from build123d import *

# Parameters (mm, degrees)
CROQUIS1_W                         = 32
CROQUIS1_H                         = 46
SALIENTE_EXTRUIR1_DEPTH            = 15
CROQUIS2_R                         = 7.5
SALIENTE_EXTRUIR2_DEPTH            = 30.8
CROQUIS3_R                         = 2.5
CROQUIS3_R_2                       = 1
CROQUIS3_R_3                       = 2.25
CROQUIS3_R_4                       = 6.25
CROQUIS3_R_5                       = 4
CROQUIS3_R_6                       = 3.958709401
CROQUIS3_R_7                       = 3.163808824
SALIENTE_EXTRUIR3_DEPTH            = 1
CORTAR_EXTRUIR1_START              = -10
CROQUIS3_3_R                       = 3.163808824
CORTAR_EXTRUIR1_DEPTH              = 10
TALADRO_DE_MARGEN_PARA_M1_41_D     = 1.8
TALADRO_DE_MARGEN_PARA_M1_41_DEPTH = 3
TALADRO_DE_MARGEN_PARA_M1_41_TIP   = 0.540774557


with BuildPart() as part:
    # Croquis1 → Saliente-Extruir1 (new body)
    with BuildSketch(Plane(origin=(0, 0, 0), x_dir=(1, 0, 0), z_dir=(0, 1, 0))):
        Rectangle(CROQUIS1_W, CROQUIS1_H)
    extrude(amount=SALIENTE_EXTRUIR1_DEPTH)

    # Croquis2 → Saliente-Extruir2 (add)
    with BuildSketch(Plane.XY.offset(23)):
        with Locations((8.5, 7.5)):
            Circle(CROQUIS2_R)
    extrude(amount=SALIENTE_EXTRUIR2_DEPTH)

    # Croquis3 → Saliente-Extruir3 (add)
    # profile 1 of 8: a face of its own
    with BuildSketch(Plane(origin=(0, 15, 0), x_dir=(1, 0, 0), z_dir=(0, 1, 0))):
        with Locations(Location((-11, 18, 0), (0, 0, 90))):
            Circle(CROQUIS3_R)
        with Locations(Location((-11, 18, 0), (0, 0, 270))):
            Circle(CROQUIS3_R_2, mode=Mode.SUBTRACT)
    # profile 2 of 8: a face of its own
    with BuildSketch(Plane(origin=(0, 15, 0), x_dir=(1, 0, 0), z_dir=(0, 1, 0))):
        with Locations(Location((11, 18, 0), (0, 0, 270))):
            Circle(CROQUIS3_R)
        with Locations(Location((11, 18, 0), (0, 0, 90))):
            Circle(CROQUIS3_R_2, mode=Mode.SUBTRACT)
    # profile 3 of 8: a face of its own
    with BuildSketch(Plane(origin=(0, 15, 0), x_dir=(1, 0, 0), z_dir=(0, 1, 0))):
        with Locations(Location((-5, -1, 0), (0, 0, 90))):
            Circle(CROQUIS3_R_3)
    # profile 4 of 8: a face of its own
    with BuildSketch(Plane(origin=(0, 15, 0), x_dir=(1, 0, 0), z_dir=(0, 1, 0))):
        with Locations(Location((5, -1, 0), (0, 0, 270))):
            Circle(CROQUIS3_R_3)
    # profile 5 of 8: a face of its own
    with BuildSketch(Plane(origin=(0, 15, 0), x_dir=(1, 0, 0), z_dir=(0, 1, 0))):
        with Locations(Location((-11, -18, 0), (0, 0, 270))):
            Circle(CROQUIS3_R)
        with Locations(Location((-11, -18, 0), (0, 0, 90))):
            Circle(CROQUIS3_R_2, mode=Mode.SUBTRACT)
    # profile 6 of 8: a face of its own
    with BuildSketch(Plane(origin=(0, 15, 0), x_dir=(1, 0, 0), z_dir=(0, 1, 0))):
        with Locations(Location((11, -18, 0), (0, 0, 90))):
            Circle(CROQUIS3_R)
        with Locations(Location((11, -18, 0), (0, 0, 270))):
            Circle(CROQUIS3_R_2, mode=Mode.SUBTRACT)
    # profile 7 of 8: a face of its own
    with BuildSketch(Plane(origin=(0, 15, 0), x_dir=(1, 0, 0), z_dir=(0, 1, 0))):
        with Locations(Location((0, 10.5, 0), (0, 0, 90))):
            Circle(CROQUIS3_R_4)
        with Locations(Location((0, 10.5, 0), (0, 0, 270))):
            Circle(CROQUIS3_R_5, mode=Mode.SUBTRACT)
    # profile 8 of 8: a face of its own
    with BuildSketch(Plane(origin=(0, 15, 0), x_dir=(1, 0, 0), z_dir=(0, 1, 0))):
        with Locations(Location((0, 10.5, 0), (0, 0, 90))):
            Circle(CROQUIS3_R_6)
        with Locations(Location((0, 10.5, 0), (0, 0, 270))):
            Circle(CROQUIS3_R_7, mode=Mode.SUBTRACT)
    extrude(amount=SALIENTE_EXTRUIR3_DEPTH)

    # Croquis3_3 → Cortar-Extruir1 (cut)
    with BuildSketch(Plane(origin=(0, 15, 0), x_dir=(1, 0, 0), z_dir=(0, 1, 0)).offset(CORTAR_EXTRUIR1_START)):
        with Locations(Location((0, 10.5, 0), (0, 0, 270))):
            Circle(CROQUIS3_3_R)
    extrude(amount=CORTAR_EXTRUIR1_DEPTH, mode=Mode.SUBTRACT)

    # Taladro de margen para M1.41
    with Locations(Plane(origin=(0, 15, 0), x_dir=(1, 0, 0), z_dir=(0, 1, 0))):
        with Locations((-14.5, 21.5), (14.5, 21.5), (-14.5, -21.5), (14.5, -21.5)):
            Hole(TALADRO_DE_MARGEN_PARA_M1_41_D / 2, depth=TALADRO_DE_MARGEN_PARA_M1_41_DEPTH)
            with Locations((0, 0, -(TALADRO_DE_MARGEN_PARA_M1_41_DEPTH + TALADRO_DE_MARGEN_PARA_M1_41_TIP / 2))):  # 118° drill point
                Cone(0, TALADRO_DE_MARGEN_PARA_M1_41_D / 2, TALADRO_DE_MARGEN_PARA_M1_41_TIP, mode=Mode.SUBTRACT)


solid = part.part
Work out the finished part from the listing and answer in its coordinate system (mm). A direction names the side the tool comes from. Round coordinates to 2 decimals unless told otherwise and drop trailing zeros. Write each loop counter-clockwise with the first axis right and the second up, starting at its lowest first coordinate (ties: lowest second). Pieces come first, ordered by that corner, then holes. Notation, with made-up numbers: (5.25, -11.75) -> (61.25, -11.75) arc R8 ccw to (61.25, -6.75) -> close; hole circle Ø5 at (60, 45). An arc over 180 degrees is marked (long way). Write each question's results on one line, items separated by ' | '.
Item 1: The mould has two halves that part along Z. Classify faces 4 (the face through (3, 16, -9)), 5 (the face through (-7, 7, 23)), 6 (the face through (14.385, 11.553, 21.394)): +Z half, -Z half, draft (parallel to the pull), parting line (faces both ways), or undercut.
Result set:
face 4: draft | face 5: +Z half | face 6: undercut
Item 2: A cutting plane is placed at B-B, the plane z = -18. Determine the outline of the cut face in (x, y), plus the area to 3 significant figures.
Result set:
outline: (-16, 0) -> (16, 0) -> (16, 15) -> (13.5, 15) -> (13.5, 16) -> (12, 16) -> (12, 15) -> (10, 15) -> (10, 16) -> (8.5, 16) -> (8.5, 15) -> (-8.5, 15) -> (-8.5, 16) -> (-10, 16) -> (-10, 15) -> (-12, 15) -> (-12, 16) -> (-13.5, 16) -> (-13.5, 15) -> (-16, 15) -> close | area: 486 mm^2
Item 3: A cutting plane is placed at A-A, the plane x = -11. Determine the outline of the cut face in (y, z).
Result set:
outline: (0, -23) -> (15, -23) -> (15, -20.5) -> (16, -20.5) -> (16, -19) -> (15, -19) -> (15, -17) -> (16, -17) -> (16, -15.5) -> (15, -15.5) -> (15, 15.5) -> (16, 15.5) -> (16, 17) -> (15, 17) -> (15, 19) -> (16, 19) -> (16, 20.5) -> (15, 20.5) -> (15, 23) -> (0, 23) -> close
Item 4: Which of the six approach directions +Z, -Z, +X, -X, +Y, -Y give full straight-line access (tool end or side, diameter ignored) to faces 1 (the face through (0, 15, 0)), 2 (the face through (14, 13, 23)), 3 (the face through (16, 7, 0))?
Result set:
face 1: +Y | face 2: +Z, +X, +Y | face 3: +Z, -Z, +X, +Y, -Y
Item 5: A cutting plane is placed at D-D, the plane z = 1. Determine the outline of the cut face in (x, y), plus the area to 3 significant figures.
Result set:
outline: (-16, 0) -> (16, 0) -> (16, 15) -> (7.25, 15) -> (7.25, 16) -> (2.75, 16) -> (2.75, 15) -> (-2.75, 15) -> (-2.75, 16) -> (-7.25, 16) -> (-7.25, 15) -> (-16, 15) -> close | area: 489 mm^2
Item 6: Find the intervals of material crossed by line 1 along X through (y, z) = (15.6, 18); line 2 along Z through (x, y) = (14.5, 13.3); line 3 along X through (y, z) = (14.5, 21.5), in increasing order. Write a range as [from, to].
Result set:
line 1: [-13.5, -12], [-10, -8.5], [8.5, 10], [12, 13.5] | line 2: [-23, -22.4], [-20.6, 20.6], [22.4, 23] | line 3: [-16, -15.4], [-13.6, 13.6], [15.4, 16]
Item 7: A cutting plane is placed at C-C, the plane y = 10. Determine the outline of the cut face in (x, z), plus the area to 3 significant figures.
Result set:
outline: (-16, -23) -> (16, -23) -> (16, 23) -> (15.57, 23) -> (15.57, 53.8) -> (1.43, 53.8) -> (1.43, 23) -> (-16, 23) -> close; hole circle Ø6.33 at (0, -10.5) | area: 1,880 mm^2
Item 8: Flat-ended cylindrical pins translate along their axes: P1, Ø1.8, axis at x = -11, z = -18, coming from the +Y side; P2, Ø1.4, axis at x = 14.5, z = 21.5, coming from the +Y side; P3, Ø4, axis at x = 0.5, z = 25.5, coming from the -Y side. Find the tip coordinate at first contact, or state that the pin passes through.
Result set:
P1: y = 15 | P2: y = 11.88 | P3: y = 3
